Verification items for the finished model (mm, model axes). Face numbers are marked on the shaded views. A direction names the side the tool comes from. Give positions to 0.01 mm unless a question says otherwise; leave off trailing zeros. Loops run counter-clockwise (first coordinate to the right, second up) from the corner with the lowest first, then second, coordinate; pieces in that order, holes last. Notation, with made-up numbers: M 81,69 L 91,69 A28 cw 91,97 Z; hole C 11,-38.75 d4. An arc over 180 degrees is marked long. Answer in a Markdown table with one row per item.
```python
from build123d import *

# Parameters (mm, degrees)
F0_W     = 88.9
F0_H     = 165.1
F1_DEPTH = 6.35
F2_DEPTH = 25.4
F3_DEPTH = 50.8
F4_R     = 6.34999
F5_SIZE  = 12.7


# Not quite as in the source:
# - a fillet or chamfer is up to 0.001 mm smaller than in the source, because OpenCascade refuses the exact size


with BuildPart() as f1:
    # F0 (on Top) → F1 (new body)
    with BuildSketch(Plane.XY):
        with Locations((-1.8205753744, 3.0884221945)):
            Rectangle(F0_W, F0_H)
        Polygon((-39.9205753744, 41.1884221945), (-39.9205753744, 79.2884221945), (-1.8205753744, 79.2884221945), (36.2794246256, 79.2884221945), (36.2794246256, -35.0115778055), (36.2794246256, -73.1115778055), (-1.8205753744, -73.1115778055), (-39.9205753744, -73.1115778055), align=None, mode=Mode.SUBTRACT)
    extrude(amount=F1_DEPTH)

    # F0 (on Top) → F2 (join)
    with BuildSketch(Plane.XY):
        with BuildLine():
            Line((36.2794246256, 79.2884221945), (-1.8205753744, 79.2884221945))
            Line((-1.8205753744, 79.2884221945), (-1.8205753744, 53.8884221945))
            ThreePointArc((-1.8205753744, 53.8884221945), (-5.5403192533, 44.9081660734), (-14.5205753744, 41.1884221945))
            Line((-14.5205753744, 41.1884221945), (-39.9205753744, 41.1884221945))
            Line((-39.9205753744, 41.1884221945), (-39.9205753744, -73.1115778055))
            Line((-39.9205753744, -73.1115778055), (-1.8205753744, -73.1115778055))
            Line((-1.8205753744, -73.1115778055), (-1.8205753744, -47.7115778055))
            ThreePointArc((-1.8205753744, -47.7115778055), (1.8991685046, -38.7313216844), (10.8794246256, -35.0115778055))
            Line((10.8794246256, -35.0115778055), (36.2794246256, -35.0115778055))
            Line((36.2794246256, -35.0115778055), (36.2794246256, 79.2884221945))
        make_face()
    extrude(amount=F2_DEPTH)

    # F0 (on Top) → F3 (join)
    with BuildSketch(Plane.XY):
        with BuildLine():
            Line((-1.8205753744, 79.2884221945), (-39.9205753744, 79.2884221945))
            Line((-39.9205753744, 79.2884221945), (-39.9205753744, 41.1884221945))
            Line((-39.9205753744, 41.1884221945), (-14.5205753744, 41.1884221945))
            ThreePointArc((-14.5205753744, 41.1884221945), (-5.5403192533, 44.9081660734), (-1.8205753744, 53.8884221945))
            Line((-1.8205753744, 53.8884221945), (-1.8205753744, 79.2884221945))
        make_face()
        with BuildLine():
            Line((36.2794246256, -73.1115778055), (36.2794246256, -35.0115778055))
            Line((36.2794246256, -35.0115778055), (10.8794246256, -35.0115778055))
            ThreePointArc((10.8794246256, -35.0115778055), (1.8991685046, -38.7313216844), (-1.8205753744, -47.7115778055))
            Line((-1.8205753744, -47.7115778055), (-1.8205753744, -73.1115778055))
            Line((-1.8205753744, -73.1115778055), (36.2794246256, -73.1115778055))
        make_face()
    extrude(amount=F3_DEPTH)

    # F4 (radius 6.35 in the source; OpenCascade refuses exactly that, so slightly less here)
    f4_edges = [f1.edges().sort_by_distance(p)[0] for p in [
        (-46.270575, 3.088422, 6.35),
        (-1.820575, -79.461578, 6.35),
        (42.629425, 3.088422, 6.35),
        (-1.820575, 85.638422, 6.35),
    ]]
    fillet(f4_edges, radius=F4_R)

    # F5
    f5_edges = [f1.edges().sort_by_distance(p)[0] for p in [
        (17.229425, -73.111578, 50.8),
        (36.279425, -54.061578, 50.8),
        (-39.920575, 60.238422, 50.8),
        (-20.870575, 79.288422, 50.8),
        (-39.920575, -15.961578, 25.4),
        (-20.870575, -73.111578, 25.4),
        (36.279425, 22.138422, 25.4),
        (17.229425, 79.288422, 25.4),
    ]]
    chamfer(f5_edges, length=F5_SIZE)


solid = f1.part
```
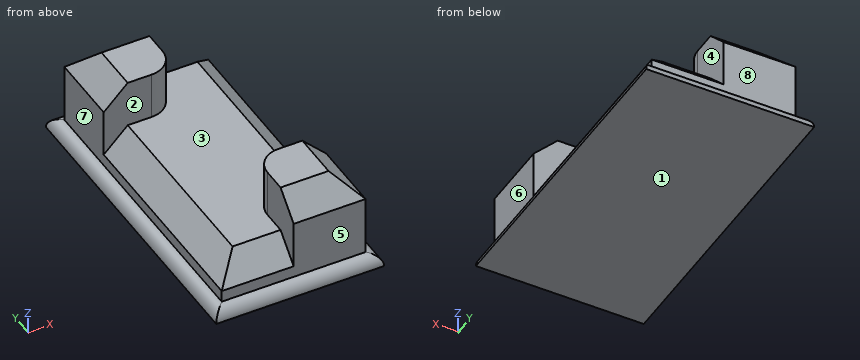
Item 1: Go/stop test with flat-tipped pins: pin 1 (3 mm diameter, centred on x = -21, z = 40, fed in from +Y); pin 2 (4 mm diameter, centred on y = -21, z = 27, fed in from +X); pin 3 (12.5 mm diameter, centred on y = 70.5, z = 35.5, fed in from +X). Record where each tip stops, or that it passes through.
Reported:
| item | result |
|---|---|
| pin 1 | stops at y = 78.89 |
| pin 2 | stops at x = 23.98 |
| pin 3 | stops at x = -1.82 |
Item 2: Sectioned sample at A-A (z = 31.5). Record the cut outline in (x, y).
Reported:
| item | result |
|---|---|
| outline | M -39.92,41.19 L -14.52,41.19 A12.7 ccw -1.82,53.89 L -1.82,79.29 L -39.92,79.29 Z; M -1.82,-73.11 L 36.28,-73.11 L 36.28,-35.01 L 10.88,-35.01 A12.7 ccw -1.82,-47.71 Z |
Item 3: Release check for a two-part mould opening along Z. For the marked faces 1, 2 and 3 record: released by +Z, released by -Z, zero draft, split by the parting line, or undercut.
Reported:
| item | result |
|---|---|
| face 1 | released by -Z |
| face 2 | zero draft |
| face 3 | released by +Z |
Item 4: Scan lines: L1, parallel to X at y = 74, z = 33; L2, parallel to X at y = 3, z = 11; L3, parallel to Z at x = -24.5, y = -23. Record each from-to range of solid material in increasing order. Write a range as [from, to].
Reported:
| item | result |
|---|---|
| L1 | x = [-39.92, -1.82] |
| L2 | x = [-39.92, 36.28] |
| L3 | z = [0, 25.4] |
Item 5: Tool access check on the marked faces 4, 5, 6, 7 and 8. Record the directions out of +Z, -Z, +X, -X, +Y, -Y that give a thin tool (end or side, any length) a straight path to the whole face; none if there is none.
Reported:
| item | result |
|---|---|
| face 4 | +Z, +X, +Y |
| face 5 | +Z, +X, -X, -Y |
| face 6 | +Z, +X, +Y, -Y |
| face 7 | +Z, -X, +Y, -Y |
| face 8 | +Z, +X, -X, +Y |
Item 6: Sectioned sample at D-D (z = 16). Record the cut outline in (x, y).
Reported:
| item | result |
|---|---|
| outline | M -39.92,41.19 L -36.62,41.19 L -36.62,-69.81 L -1.82,-69.81 L -1.82,-73.11 L 36.28,-73.11 L 36.28,-35.01 L 32.98,-35.01 L 32.98,75.99 L -1.82,75.99 L -1.82,79.29 L -39.92,79.29 Z |
